from build123d import *

# Parameters (mm, degrees)
BOSS_EXTRUDE1_DEPTH = 5
SKETCH3_R           = 2.5
CUT_EXTRUDE1_DEPTH  = 162.241436536
BOSS_EXTRUDE2_DEPTH = 20
BOSS_EXTRUDE3_DEPTH = 5


with BuildPart() as part:
    # Sketch1 → Boss-Extrude1 (new body)
    with BuildSketch(Plane(origin=(0, 0, 0), x_dir=(1, 0, 0), z_dir=(0, 1, 0))):
        Polygon((-75, 106.6), (-75, -106.6), (-98.766968108, -111.353393622), (-98.766968108, -127.353393622), (-86.766968108, -127.353393622), (-75, -125), (0, -110), (75, -125), (86.766968108, -127.353393622), (98.766968108, -127.353393622), (98.766968108, -111.353393622), (75, -106.6), (75, 106.6), (98.766968108, 111.353393622), (98.766968108, 127.353393622), (86.766968108, 127.353393622), (75, 125), (0, 110), (-75, 125), (-86.766968108, 127.353393622), (-98.766968108, 127.353393622), (-98.766968108, 111.353393622), align=None)
    extrude(amount=BOSS_EXTRUDE1_DEPTH)

    # Sketch3 → Cut-Extrude1 (cut, through all)
    with BuildSketch(Plane(origin=(0, 5, 0), x_dir=(1, 0, 0), z_dir=(0, 1, 0))):
        Polygon((-73, 106.6), (-73, -106.6), (-73, -122.560392195), (0, -107.960392195), (73, -122.560392195), (73, -106.6), (73, 106.6), (73, 122.560392195), (0, 107.960392195), (-73, 122.560392195), align=None)
        with Locations(Location((-82.176846176, -117.235369235, 0), (0, 0, 270))):
            Circle(SKETCH3_R)
        with Locations(Location((82.176846176, -117.235369235, 0), (0, 0, 270))):
            Circle(SKETCH3_R)
        with Locations(Location((-82.176846176, 117.235369235, 0), (0, 0, 270))):
            Circle(SKETCH3_R)
        with Locations(Location((82.176846176, 117.235369235, 0), (0, 0, 270))):
            Circle(SKETCH3_R)
    extrude(amount=-CUT_EXTRUDE1_DEPTH, mode=Mode.SUBTRACT)

    # Sketch4 → Boss-Extrude2 (add)
    with BuildSketch(Plane(origin=(0, 5, 0), x_dir=(1, 0, 0), z_dir=(0, 1, 0))):
        Polygon((-75, 125), (-75, -125), (0, -110), (75, -125), (75, 125), (0, 110), align=None)
        Polygon((0, -107.960392195), (73, -122.560392195), (73, 122.560392195), (0, 107.960392195), (-73, 122.560392195), (-73, -122.560392195), align=None, mode=Mode.SUBTRACT)
    extrude(amount=BOSS_EXTRUDE2_DEPTH)

    # Sketch5 → Boss-Extrude3 (add)
    with BuildSketch(Plane(origin=(0, 25, 0), x_dir=(1, 0, 0), z_dir=(0, 1, 0))):
        Polygon((75, 125), (0, 110), (-75, 125), (-75, -125), (0, -110), (75, -125), align=None)
    extrude(amount=-BOSS_EXTRUDE3_DEPTH)


solid = part.part
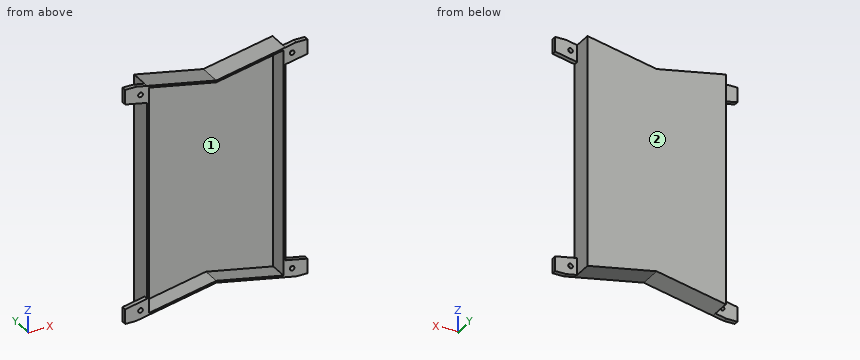
Check sheet for the modelled part. Datum: model origin and axes. Units: mm. Face numbers are marked on the shaded views. Give positions to 0.01 mm unless a question says otherwise; leave off trailing zeros. Loops run counter-clockwise (first coordinate to the right, second up) from the corner with the lowest first, then second, coordinate; pieces in that order, holes last. Notation, with made-up numbers: M -23.75,38 L -0.75,38 A8 ccw -0.75,49 Z; hole C 36.25,-37.5 d5. An arc over 180 degrees is marked long. Return JSON: item names as keys, results as strings. Group by question number.
1. Go/stop test with flat-tipped pins: pin 1 (8 mm diameter, centred on y = 17.5, z = -15, fed in from -X); pin 2 (4 mm diameter, centred on x = -82.18, z = 117.24, fed in from -Y); pin 3 (12 mm diameter, centred on x = 2.5, y = 10, fed in from -Z); pin 4 (6 mm diameter, centred on x = -87, z = -113, fed in from +Y). Record where each tip stops, or that it passes through.
2. Mould release check, pull along Z, two halves, no side actions. Record for the marked faces 1 and 2: released by +Z, released by -Z, zero draft, split by the parting line, or undercut.
3. Cross-section at C-C on z = 77.5. Record the boundary of the cut face in (x, y).
4. Cross-section at B-B on x = -67. Record the boundary of the cut face in (y, z).
5. Thickness scan on L1, parallel to X at y = 15.75, z = 51; L2, parallel to Y at x = -49, z = 66.5; L3, parallel to Z at x = 79, y = 4.5. Record the ranges inside material, lowest first.
6. Cross-section at A-A on y = 13. Record the boundary of the cut face in (x, z), plus the area to 3 significant figures.
Return value:
{
 "1": {"pin 1": "x = -75", "pin 2": "through", "pin 3": "z = -111.7", "pin 4": "y = 5"},
 "2": {"face 1": "undercut", "face 2": "zero draft"},
 "3": {"outline": "M -75,0 L -73,0 L -73,20 L 73,20 L 73,0 L 75,0 L 75,25 L -75,25 Z"},
 "4": {"outline": "M 0,-123.4 L 25,-123.4 L 25,123.4 L 0,123.4 L 0,121.36 L 20,121.36 L 20,-121.36 L 0,-121.36 Z"},
 "5": {"L1": "-75 to -73, 73 to 75", "L2": "20 to 25", "L3": "-125.8 to -107.4, 107.4 to 125.8"},
 "6": {"outline": "M -75,-125 L 0,-110 L 75,-125 L 75,125 L 0,110 L -75,125 Z; hole M -73,-122.56 L 0,-107.96 L 73,-122.56 L 73,122.56 L 0,107.96 L -73,122.56 Z", "area": "1,590 mm^2"}
}
